Read the model definition and answer for the solid it produces. Units are mm, in the model's axes. Round coordinates to 2 decimals unless told otherwise and drop trailing zeros. Write each loop counter-clockwise with the first axis right and the second up, starting at its lowest first coordinate (ties: lowest second). Pieces come first, ordered by that corner, then holes. Notation, with made-up numbers: (11.5, 89.5) -> (31.5, 89.5) arc R15 ccw to (31.5, 106.5) -> close; hole circle Ø7 at (-19.5, -33). An arc over 180 degrees is marked (long way). Return JSON: item names as keys, results as strings.
from build123d import *

# Parameters (mm, degrees)
F0_R       = 1.98755
F0_R_2     = 2.59715
F1_DEPTH   = 1.7272
F2_R       = 0.381
F3_R       = 0.381
F4_SIZE2   = 0.3299556788
F4_SIZE    = 0.1905
F4_2_SIZE2 = 0.3299556788
F4_2_SIZE  = 0.1905
F5_SIZE2   = 0.2859615883
F5_SIZE    = 0.1651
F5_2_SIZE2 = 0.2859615883
F5_2_SIZE  = 0.1651


with BuildPart() as f1:
    # F0 (on Front) → F1 (new body, symmetric)
    with BuildSketch(Plane.XZ):
        with BuildLine():
            ThreePointArc((4.6498341341, -0.4707223022), (0, 4.6736), (-4.6498341341, -0.4707223022))
            Line((-4.6498341341, -0.4707223022), (-3.9422506789, -7.4602906475))
            ThreePointArc((-3.9422506789, -7.4602906475), (0, -11.0236), (3.9422506789, -7.4602906475))
            Line((3.9422506789, -7.4602906475), (4.6498341341, -0.4707223022))
        make_face()
        with Locations((0, -7.0612)):
            Circle(F0_R, mode=Mode.SUBTRACT)
        Circle(F0_R_2, mode=Mode.SUBTRACT)
    extrude(amount=F1_DEPTH, both=True)

    # F2
    f2_edges = [f1.edges().sort_by_distance(p)[0] for p in [
        (4.296042, -1.7272, -3.965506),
        (0, -1.7272, 4.6736),
        (-4.296042, -1.7272, -3.965506),
        (0, -1.7272, -11.0236),
    ]]
    fillet(f2_edges, radius=F2_R)

    # F3
    f3_edges = [f1.edges().sort_by_distance(p)[0] for p in [
        (4.296042, 1.7272, -3.965506),
        (0, 1.7272, 4.6736),
        (-4.296042, 1.7272, -3.965506),
        (0, 1.7272, -11.0236),
    ]]
    fillet(f3_edges, radius=F3_R)

    # F4
    f4_edges = [f1.edges().sort_by_distance(p)[0] for p in [
        (-2.59715, -1.7272, 0),
    ]]
    f4_side = f1.faces().sort_by_distance((0, -1.7272, -3.137355))[0]
    chamfer(f4_edges, length=F4_SIZE, length2=F4_SIZE2, reference=f4_side)

    # F4#2
    f4_2_edges = [f1.edges().sort_by_distance(p)[0] for p in [
        (-2.59715, 1.7272, 0),
    ]]
    f4_2_side = f1.faces().sort_by_distance((0, 1.7272, -3.137355))[0]
    chamfer(f4_2_edges, length=F4_2_SIZE, length2=F4_2_SIZE2, reference=f4_2_side)

    # F5
    f5_edges = [f1.edges().sort_by_distance(p)[0] for p in [
        (-1.98755, -1.7272, -7.0612),
    ]]
    f5_side = f1.faces().sort_by_distance((0, -1.7272, -3.285713))[0]
    chamfer(f5_edges, length=F5_SIZE, length2=F5_SIZE2, reference=f5_side)

    # F5#2
    f5_2_edges = [f1.edges().sort_by_distance(p)[0] for p in [
        (-1.98755, 1.7272, -7.0612),
    ]]
    f5_2_side = f1.faces().sort_by_distance((0, 1.7272, -3.285713))[0]
    chamfer(f5_2_edges, length=F5_2_SIZE, length2=F5_2_SIZE2, reference=f5_2_side)


solid = f1.part
Item 1: Straight lines are drawn through the part: L1, parallel to Z at x = 0, y = -0.35; L2, parallel to Z at x = -0.75, y = -1; L3, parallel to X at y = -1.5, z = 0. For each, find the intervals that lie inside material, in ascending order. Write a range as [from, to].
Worked answers:
{"L1": "z = [-11.02, -9.05], [-5.07, -2.6], [2.6, 4.67]", "L2": "z = [-10.95, -8.9], [-5.22, -2.49], [2.49, 4.61]", "L3": "x = [-4.64, -2.66], [2.66, 4.64]"}
Item 2: Section B-B (y = 0.2) is taken. Give the vertices of the cut face in (x, z), then the cut area to 3 significant figures.
Worked answers:
{"outline": "(-4.65, -0.47) -> (-3.94, -7.46) arc R3.96 ccw to (3.94, -7.46) -> (4.65, -0.47) arc R4.67 ccw (long way) to start; hole circle Ø5.19 at (0, 0); hole circle Ø3.98 at (0, -7.06)", "area": "86.7 mm2"}
Item 3: Section A-A (x = 0) is taken. Give the vertices of the cut face in (y, z).
Worked answers:
{"outline": "(-1.73, -10.64) arc R0.38 ccw to (-1.35, -11.02) -> (1.35, -11.02) arc R0.38 ccw to (1.73, -10.64) -> (1.73, -9.21) -> (1.44, -9.05) -> (-1.44, -9.05) -> (-1.73, -9.21) -> close; (-1.73, -4.91) -> (-1.44, -5.07) -> (1.44, -5.07) -> (1.73, -4.91) -> (1.73, -2.79) -> (1.4, -2.6) -> (-1.4, -2.6) -> (-1.73, -2.79) -> close; (-1.73, 2.79) -> (-1.4, 2.6) -> (1.4, 2.6) -> (1.73, 2.79) -> (1.73, 4.29) arc R0.38 ccw to (1.35, 4.67) -> (-1.35, 4.67) arc R0.38 ccw to (-1.73, 4.29) -> close"}
Item 4: Section C-C (x = 1.5) is taken. State how many separate pieces and enclosed holes the cut face has, then the cut area to 3 significant figures.
Worked answers:
{"separate pieces": "3", "enclosed holes": "0", "area": "28.3 mm2"}
Item 5: Flat-ended cylindrical pins translate along their axes: pin 1 (1 mm diameter, centred on x = -1, z = -8.5, fed in from +Y); pin 2 (1 mm diameter, centred on y = 1.5, z = -4, fed in from -X); pin 3 (4 mm diameter, centred on x = 0, z = 0, fed in from -Y). Find the tip coordinate at first contact, or state that the pin passes through.
Worked answers:
{"pin 1": "stops at y = 1.73", "pin 2": "stops at x = -4.34", "pin 3": "passes through"}
